For this review, use the dimensioned drawing (mm, ordinates from the lowest corner) and the shaded views. Coordinates: 2 decimals unless noted, no trailing zeros. Loops run counter-clockwise (first coordinate to the right, second up) from the corner with the lowest first, then second, coordinate; pieces in that order, holes last. Notation, with made-up numbers: M 46,76.25 L 89,76.25 A25 cw 89,103.25 Z; hole C 77,75.5 d10. An arc over 180 degrees is marked long. One line per item, written item: value.
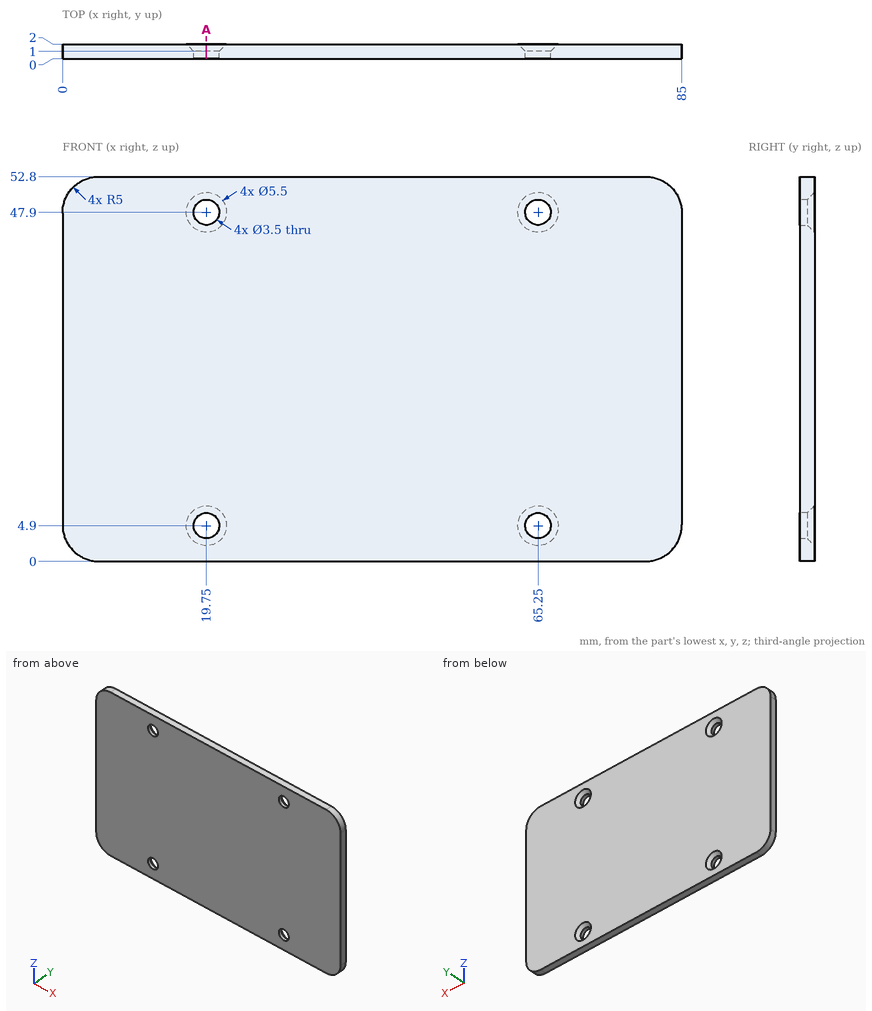
(1) Insertion check: pin 1 (4 mm diameter, centred on x = 43.5, z = 42, fed in from -Y). The pin has a flat end and moves straight along its axis. Give the tip position at first contact, or say it passes through.
Reply:
pin 1: stops at y = 0
(2) We need section A-A on x = 19.75. State the section outline as (y, z) points.
Reply:
outline: M 0,0 L 2,0 L 2,2.15 L 1,3.15 L 0,3.15 Z; M 0,6.65 L 1,6.65 L 2,7.65 L 2,45.15 L 1,46.15 L 0,46.15 Z; M 0,49.65 L 1,49.65 L 2,50.65 L 2,52.8 L 0,52.8 Z
(3) To check wall thickness, follow line 1 along Z through (x, y) = (65.25, 0.7); line 2 along X through (y, z) = (0.2, 47.9); line 3 along X through (y, z) = (1.7, 50). State the ranges of each line that lie inside material, in increasing order. Write a range as [from, to].
Reply:
line 1: z = [0, 3.15], [6.65, 46.15], [49.65, 52.8]
line 2: x = [0, 18], [21.5, 63.5], [67, 85]
line 3: x = [0.51, 18.49], [21.01, 63.99], [66.51, 84.49]
